from build123d import *

# Parameters (mm, degrees)
SKETCH1_W           = 76.72
SKETCH1_H           = 26.686
BOSS_EXTRUDE1_DEPTH = 15
SKETCH2_W           = 11
SKETCH2_H           = 5
CUT_EXTRUDE1_DEPTH  = 69.000448499
SKETCH3_R           = 1.5
CUT_EXTRUDE2_DEPTH  = 25
CUT_EXTRUDE3_DEPTH  = 3
CUT_EXTRUDE5_DEPTH  = 7
FILLET1_R           = 5


with BuildPart() as part:
    # Sketch1 → Boss-Extrude1 (new body)
    with BuildSketch(Plane.XY):
        with Locations((22.36, 8.343)):
            Rectangle(SKETCH1_W, SKETCH1_H)
        Polygon((0, 0), (0, 12), (3.02, 16.686), (5.22, 16.686), (8.24, 12), (8.24, 0), align=None, mode=Mode.SUBTRACT)
        Polygon((23.46, 16.686), (26.48, 12), (26.48, 0), (18.24, 0), (18.24, 12), (21.26, 16.686), align=None, mode=Mode.SUBTRACT)
        Polygon((41.7, 16.686), (44.72, 12), (44.72, 0), (36.48, 0), (36.48, 12), (39.5, 16.686), align=None, mode=Mode.SUBTRACT)
    extrude(amount=BOSS_EXTRUDE1_DEPTH)

    # Sketch2 → Cut-Extrude1 (cut, through all)
    with BuildSketch(Plane(origin=(0, -5, 0), x_dir=(-1, 0, 0), z_dir=(0, -1, 0))):
        with Locations((10.5, -12.5)):
            Rectangle(SKETCH2_W, SKETCH2_H)
        with Locations((-55.22, -12.5)):
            Rectangle(SKETCH2_W, SKETCH2_H)
    extrude(amount=-CUT_EXTRUDE1_DEPTH, mode=Mode.SUBTRACT)

    # Sketch3 → Cut-Extrude2 (cut)
    with BuildSketch(Plane.XY.offset(10)):
        with Locations((-10.5, 7.331502285)):
            Circle(SKETCH3_R)
        with Locations((55.22, 7.331502285)):
            Circle(SKETCH3_R)
    extrude(amount=-CUT_EXTRUDE2_DEPTH, mode=Mode.SUBTRACT)

    # Sketch4 → Cut-Extrude3 (cut)
    with BuildSketch(Plane.XY.offset(10)):
        Polygon((-10.5, 10.651266332), (-13.375, 8.991384309), (-13.375, 5.671620261), (-10.5, 4.011738237), (-7.625, 5.671620261), (-7.625, 8.991384309), align=None)
        Polygon((55.22, 10.651266332), (52.345, 8.991384309), (52.345, 5.671620261), (55.22, 4.011738237), (58.095, 5.671620261), (58.095, 8.991384309), align=None)
    extrude(amount=-CUT_EXTRUDE3_DEPTH, mode=Mode.SUBTRACT)

    # Sketch7 → Cut-Extrude5 (cut)
    with BuildSketch(Plane(origin=(0, 0, 0), x_dir=(-1, 0, 0), z_dir=(0, 0, -1))):
        Polygon((0, 0), (-12.36, 0), (-12.36, -5), (-32.36, -5), (-32.36, 0), (-44.72, 0), (-44.72, 16.686), (0, 16.686), align=None)
    extrude(amount=-CUT_EXTRUDE5_DEPTH, mode=Mode.SUBTRACT)

    # Fillet1
    # the kernel refuses this fillet: 5 mm, written as the material it adds along each edge
    with BuildSketch(Plane(origin=(49.72, -5, 10), x_dir=(0, 0, 1), z_dir=(0, 1, 0))) as fillet1_piece_1_section:
        with BuildLine():
            CenterArc((FILLET1_R, FILLET1_R), FILLET1_R, 180, 90)
            Line((0, FILLET1_R), (0, 0))
            Line((0, 0), (FILLET1_R, 0))
        make_face()
    fillet1_piece_1 = extrude(amount=26.686, mode=Mode.PRIVATE)
    fillet1_piece_1 = split(fillet1_piece_1, bisect_by=Plane(origin=(52.345, 0.855809372, 11.280904263), z_dir=(-1, 0, 0)), keep=Keep.TOP, mode=Mode.PRIVATE)
    fillet1_piece_1 = split(fillet1_piece_1, bisect_by=Plane(origin=(53.079309625, 5.247666401, 11.280904263), z_dir=(-0.5000000000000012, -0.866025403784438, 0)), keep=Keep.TOP, mode=Mode.PRIVATE)
    add(fillet1_piece_1)
    with BuildSketch(Plane(origin=(49.72, -5, 10), x_dir=(0, 0, 1), z_dir=(0, 1, 0))) as fillet1_piece_2_section:
        with BuildLine():
            CenterArc((FILLET1_R, FILLET1_R), FILLET1_R, 180, 90)
            Line((0, FILLET1_R), (0, 0))
            Line((0, 0), (FILLET1_R, 0))
        make_face()
    fillet1_piece_2 = extrude(amount=26.686, mode=Mode.PRIVATE)
    fillet1_piece_2 = split(fillet1_piece_2, bisect_by=Plane(origin=(52.345, 0.113882783, 10.103766802), z_dir=(1, 0, 0)), keep=Keep.TOP, mode=Mode.PRIVATE)
    fillet1_piece_2 = split(fillet1_piece_2, bisect_by=Plane(origin=(55.328155085, 3.94929487, 10.103766802), z_dir=(-0.5000000000000012, -0.866025403784438, 0)), keep=Keep.TOP, mode=Mode.PRIVATE)
    add(fillet1_piece_2)
    with BuildSketch(Plane(origin=(49.72, -5, 10), x_dir=(0, 0, 1), z_dir=(0, 1, 0))) as fillet1_piece_3_section:
        with BuildLine():
            CenterArc((FILLET1_R, FILLET1_R), FILLET1_R, 180, 90)
            Line((0, FILLET1_R), (0, 0))
            Line((0, 0), (FILLET1_R, 0))
        make_face()
    fillet1_piece_3 = extrude(amount=26.686, mode=Mode.PRIVATE)
    fillet1_piece_3 = split(fillet1_piece_3, bisect_by=Plane(origin=(50.660222367, 8.018677488, 10.86123456), z_dir=(0.5000000000000002, -0.8660254037844386, 0)), keep=Keep.TOP, mode=Mode.PRIVATE)
    fillet1_piece_3 = split(fillet1_piece_3, bisect_by=Plane(origin=(52.345, 7.331502285, 10.86123456), z_dir=(-1, 0, 0)), keep=Keep.TOP, mode=Mode.PRIVATE)
    fillet1_piece_3 = split(fillet1_piece_3, bisect_by=Plane(origin=(50.660222367, 6.644327081, 10.86123456), z_dir=(0.5000000000000012, 0.866025403784438, 0)), keep=Keep.TOP, mode=Mode.PRIVATE)
    add(fillet1_piece_3)
    with BuildSketch(Plane(origin=(49.72, -5, 10), x_dir=(0, 0, 1), z_dir=(0, 1, 0))) as fillet1_piece_4_section:
        with BuildLine():
            CenterArc((FILLET1_R, FILLET1_R), FILLET1_R, 180, 90)
            Line((0, FILLET1_R), (0, 0))
            Line((0, 0), (FILLET1_R, 0))
        make_face()
    fillet1_piece_4 = extrude(amount=26.686, mode=Mode.PRIVATE)
    fillet1_piece_4 = split(fillet1_piece_4, bisect_by=Plane(origin=(53.520712077, 9.670181993, 11.277716929), z_dir=(-0.5000000000000002, 0.8660254037844386, 0)), keep=Keep.TOP, mode=Mode.PRIVATE)
    fillet1_piece_4 = split(fillet1_piece_4, bisect_by=Plane(origin=(52.345, 14.819818281, 11.277716929), z_dir=(-1, 0, 0)), keep=Keep.TOP, mode=Mode.PRIVATE)
    add(fillet1_piece_4)
    with BuildSketch(Plane(origin=(49.72, -5, 10), x_dir=(0, 0, 1), z_dir=(0, 1, 0))) as fillet1_piece_5_section:
        with BuildLine():
            CenterArc((FILLET1_R, FILLET1_R), FILLET1_R, 180, 90)
            Line((0, FILLET1_R), (0, 0))
            Line((0, 0), (FILLET1_R, 0))
        make_face()
    fillet1_piece_5 = extrude(amount=26.686, mode=Mode.PRIVATE)
    fillet1_piece_5 = split(fillet1_piece_5, bisect_by=Plane(origin=(55.769242126, 10.968371422, 10.103260702), z_dir=(-0.5000000000000002, 0.8660254037844386, 0)), keep=Keep.TOP, mode=Mode.PRIVATE)
    fillet1_piece_5 = split(fillet1_piece_5, bisect_by=Plane(origin=(52.345, 15.561640812, 10.103260702), z_dir=(1, 0, 0)), keep=Keep.TOP, mode=Mode.PRIVATE)
    add(fillet1_piece_5)
    with BuildSketch(Plane(origin=(-5, -5, 10), x_dir=(-1, 0, 0), z_dir=(0, 1, 0))) as fillet1_piece_6_section:
        with BuildLine():
            CenterArc((FILLET1_R, FILLET1_R), FILLET1_R, 180, 90)
            Line((0, FILLET1_R), (0, 0))
            Line((0, 0), (FILLET1_R, 0))
        make_face()
    fillet1_piece_6 = extrude(amount=26.686, mode=Mode.PRIVATE)
    fillet1_piece_6 = split(fillet1_piece_6, bisect_by=Plane(origin=(-10.608155085, 3.94929487, 10.103766802), z_dir=(0.5000000000000003, -0.8660254037844387, 0)), keep=Keep.TOP, mode=Mode.PRIVATE)
    fillet1_piece_6 = split(fillet1_piece_6, bisect_by=Plane(origin=(-7.625, 0.113882783, 10.103766802), z_dir=(-1, 0, 0)), keep=Keep.TOP, mode=Mode.PRIVATE)
    add(fillet1_piece_6)
    with BuildSketch(Plane(origin=(-5, -5, 10), x_dir=(-1, 0, 0), z_dir=(0, 1, 0))) as fillet1_piece_7_section:
        with BuildLine():
            CenterArc((FILLET1_R, FILLET1_R), FILLET1_R, 180, 90)
            Line((0, FILLET1_R), (0, 0))
            Line((0, 0), (FILLET1_R, 0))
        make_face()
    fillet1_piece_7 = extrude(amount=26.686, mode=Mode.PRIVATE)
    fillet1_piece_7 = split(fillet1_piece_7, bisect_by=Plane(origin=(-8.359309625, 5.247666401, 11.280904263), z_dir=(0.5000000000000003, -0.8660254037844387, 0)), keep=Keep.TOP, mode=Mode.PRIVATE)
    fillet1_piece_7 = split(fillet1_piece_7, bisect_by=Plane(origin=(-7.625, 0.855809372, 11.280904263), z_dir=(1, 0, 0)), keep=Keep.TOP, mode=Mode.PRIVATE)
    add(fillet1_piece_7)
    with BuildSketch(Plane(origin=(-5, -5, 10), x_dir=(-1, 0, 0), z_dir=(0, 1, 0))) as fillet1_piece_8_section:
        with BuildLine():
            CenterArc((FILLET1_R, FILLET1_R), FILLET1_R, 180, 90)
            Line((0, FILLET1_R), (0, 0))
            Line((0, 0), (FILLET1_R, 0))
        make_face()
    fillet1_piece_8 = extrude(amount=26.686, mode=Mode.PRIVATE)
    fillet1_piece_8 = split(fillet1_piece_8, bisect_by=Plane(origin=(-5.940222366, 6.644327081, 10.861234561), z_dir=(-0.5000000000000003, 0.8660254037844387, 0)), keep=Keep.TOP, mode=Mode.PRIVATE)
    fillet1_piece_8 = split(fillet1_piece_8, bisect_by=Plane(origin=(-7.625, 7.331502285, 10.861234561), z_dir=(1, 0, 0)), keep=Keep.TOP, mode=Mode.PRIVATE)
    fillet1_piece_8 = split(fillet1_piece_8, bisect_by=Plane(origin=(-5.940222366, 8.018677488, 10.861234561), z_dir=(-0.49999999999999967, -0.8660254037844388, 0)), keep=Keep.TOP, mode=Mode.PRIVATE)
    add(fillet1_piece_8)
    with BuildSketch(Plane(origin=(-5, -5, 10), x_dir=(-1, 0, 0), z_dir=(0, 1, 0))) as fillet1_piece_9_section:
        with BuildLine():
            CenterArc((FILLET1_R, FILLET1_R), FILLET1_R, 180, 90)
            Line((0, FILLET1_R), (0, 0))
            Line((0, 0), (FILLET1_R, 0))
        make_face()
    fillet1_piece_9 = extrude(amount=26.686, mode=Mode.PRIVATE)
    fillet1_piece_9 = split(fillet1_piece_9, bisect_by=Plane(origin=(-7.625, 15.561640812, 10.103260702), z_dir=(-1, 0, 0)), keep=Keep.TOP, mode=Mode.PRIVATE)
    fillet1_piece_9 = split(fillet1_piece_9, bisect_by=Plane(origin=(-11.049242126, 10.968371422, 10.103260702), z_dir=(0.49999999999999967, 0.8660254037844388, 0)), keep=Keep.TOP, mode=Mode.PRIVATE)
    add(fillet1_piece_9)
    with BuildSketch(Plane(origin=(-5, -5, 10), x_dir=(-1, 0, 0), z_dir=(0, 1, 0))) as fillet1_piece_10_section:
        with BuildLine():
            CenterArc((FILLET1_R, FILLET1_R), FILLET1_R, 180, 90)
            Line((0, FILLET1_R), (0, 0))
            Line((0, 0), (FILLET1_R, 0))
        make_face()
    fillet1_piece_10 = extrude(amount=26.686, mode=Mode.PRIVATE)
    fillet1_piece_10 = split(fillet1_piece_10, bisect_by=Plane(origin=(-7.625, 14.819818281, 11.277716929), z_dir=(1, 0, 0)), keep=Keep.TOP, mode=Mode.PRIVATE)
    fillet1_piece_10 = split(fillet1_piece_10, bisect_by=Plane(origin=(-8.800712077, 9.670181993, 11.277716929), z_dir=(0.49999999999999967, 0.8660254037844388, 0)), keep=Keep.TOP, mode=Mode.PRIVATE)
    add(fillet1_piece_10)
    # the kernel refuses this fillet: 5 mm, written as the material it takes off along each edge
    with BuildSketch(Plane(origin=(60.72, -17.5, 10), x_dir=(0, 0, -1), z_dir=(0, 1, 0)), Plane(origin=(-16, -17.5, 10), x_dir=(1, 0, 0), z_dir=(0, 1, 0))) as fillet1_2_piece_1:
        with BuildLine():
            CenterArc((FILLET1_R, FILLET1_R), FILLET1_R, 180, 90)
            Line((0, FILLET1_R), (0, 0))
            Line((0, 0), (FILLET1_R, 0))
        make_face()
    extrude(amount=51.686, mode=Mode.SUBTRACT)
    with BuildSketch(Plane(origin=(73.22, 21.686, 10), x_dir=(0, 0, -1), z_dir=(-1, 0, 0)), Plane(origin=(-10, 21.686, 10), x_dir=(0, 0, -1), z_dir=(-1, 0, 0))) as fillet1_2_piece_2:
        with BuildLine():
            CenterArc((FILLET1_R, FILLET1_R), FILLET1_R, 180, 90)
            Line((0, FILLET1_R), (0, 0))
            Line((0, 0), (FILLET1_R, 0))
        make_face()
    extrude(amount=18.5, mode=Mode.SUBTRACT)
    with BuildSketch(Plane(origin=(73.22, -5, 10), x_dir=(0, 0, -1), z_dir=(-1, 0, 0)), Plane(origin=(-10, -5, 10), x_dir=(0, 0, -1), z_dir=(-1, 0, 0))) as fillet1_2_piece_3:
        with BuildLine():
            CenterArc((FILLET1_R, -FILLET1_R), FILLET1_R, 90, 90)
            Line((0, -FILLET1_R), (0, 0))
            Line((0, 0), (FILLET1_R, 0))
        make_face()
    extrude(amount=18.5, mode=Mode.SUBTRACT)
    with BuildSketch(Plane(origin=(-10, -5, 15), x_dir=(-0.8017442392976459, 0, 0.5976672776328307), z_dir=(-0.5976672776328307, 0, -0.8017442392976459))) as fillet1_2_piece_4:
        with BuildLine():
            CenterArc((5 + FILLET1_R, FILLET1_R), FILLET1_R, 180, 90)
            Line((5, FILLET1_R), (5, 0))
            Line((5, 0), (5 + FILLET1_R, 0))
        make_face()
    revolve(axis=Axis((-10, -5, 15), (0, 1, 0)), revolution_arc=233.296989237, mode=Mode.SUBTRACT)
    with BuildSketch(Plane(origin=(-10, 21.686, 15), x_dir=(0, 0, -1), z_dir=(-1, 0, 0))) as fillet1_2_piece_5:
        with BuildLine():
            CenterArc((5 + FILLET1_R, FILLET1_R), FILLET1_R, 180, 90)
            Line((5, FILLET1_R), (5, 0))
            Line((5, 0), (5 + FILLET1_R, 0))
        make_face()
    revolve(axis=Axis((-10, 21.686, 15), (0, -1, 0)), revolution_arc=233.296989237, mode=Mode.SUBTRACT)
    with BuildSketch(Plane(origin=(54.72, -5, 15), x_dir=(0, 0, -1), z_dir=(1, 0, 0))) as fillet1_2_piece_6:
        with BuildLine():
            CenterArc((5 + FILLET1_R, FILLET1_R), FILLET1_R, 180, 90)
            Line((5, FILLET1_R), (5, 0))
            Line((5, 0), (5 + FILLET1_R, 0))
        make_face()
    revolve(axis=Axis((54.72, -5, 15), (0, 1, 0)), revolution_arc=233.296989237, mode=Mode.SUBTRACT)
    with BuildSketch(Plane(origin=(54.72, 21.686, 15), x_dir=(0.8017442392976476, 0, 0.5976672776328285), z_dir=(0.5976672776328285, 0, -0.8017442392976476))) as fillet1_2_piece_7:
        with BuildLine():
            CenterArc((5 + FILLET1_R, FILLET1_R), FILLET1_R, 180, 90)
            Line((5, FILLET1_R), (5, 0))
            Line((5, 0), (5 + FILLET1_R, 0))
        make_face()
    revolve(axis=Axis((54.72, 21.686, 15), (0, -1, 0)), revolution_arc=233.296989237, mode=Mode.SUBTRACT)


solid = part.part
Read the model definition and answer for the solid it produces. Units are mm, in the model's axes. A direction names the side the tool comes from. Coordinates: 2 decimals unless noted, no trailing zeros. Loops run counter-clockwise (first coordinate to the right, second up) from the corner with the lowest first, then second, coordinate; pieces in that order, holes last. Notation, with made-up numbers: (-24.5, 11.5) -> (1.5, 11.5) arc R24 cw to (1.5, 31.5) -> close; hole circle Ø11 at (80, 22). An arc over 180 degrees is marked (long way). Write item = value, one per line. Start each with the question number.
1) Find the intervals of material crossed by L1, parallel to Y at x = -10.5, z = 4; L2, parallel to X at y = 8.5, z = 11.5; L3, parallel to Y at x = 23, z = 8.25, in increasing order. Write a range as from..to.
2) The part is cut by section A-A, the plane y = 12.75. Determine the outline of the cut face in (x, z), plus the area to 3 significant figures.
3) The mould has two halves that part along Y. Classify faces 1 (the face through (32.36, -3, 3)), 2 (the face through (52.345, 7, 9)), 3 (the face through (57, -4, 8)), 4 (the face through (37.97, 14.31, 10.94)): pulls with the +Y half, pulls with the -Y half, needs draft (parallel to the pull), parting line crosses it, or undercut.
4) For faces 5 (the face through (12.36, -2, 3)), 6 (the face through (44, 15, 7)), 7 (the face through (43.189, 14.376, 10.944)), 8 (the face through (-11.958, 4.853, 8.521)), 9 (the face through (16, 9, 15)), determine the directions among +Z, -Z, +X, -X, +Y, -Y from which every point of the face is accessible in a straight line to the end or side of a thin tool.
5) Given P1, Ø1.9, axis at y = 7.5, z = 7.5, coming from the +X side; P2, Ø11, axis at x = 28, y = 4, coming from the -Z side; P3, Ø6, axis at y = 13, z = 11, coming from the +X side; P4, Ø1.8, axis at x = 55.22, y = 7.33, coming from the +Z side, each flat-ended and moving along its own axis, determine where each tip first touches the part or whether it passes through.
6) The part is cut by section C-C, the plane z = 13.75. State how many separate pieces and enclosed holes the cut face has, plus the area to 3 significant figures.
7) The part is cut by section B-B, the plane z = 1.25. Determine the outline of the cut face in (x, y), plus the area to 3 significant figures.
Result:
q1.L1 = -5..5.83, 8.83..21.69
q1.L2 = -6.43..0, 8.24..18.24, 26.48..36.48, 44.72..51.15
q1.L3 = -5..0, 16.69..21.69
q2.outline = (-16, 0) -> (0, 0) -> (0, 7) -> (0.48, 7) -> (0.48, 15) -> (-5, 15) arc R5 cw to (-10, 10) -> (-11, 10) arc R5 ccw to (-16, 5) -> close; (7.76, 7) -> (18.72, 7) -> (18.72, 15) -> (7.76, 15) -> close; (26, 7) -> (36.96, 7) -> (36.96, 15) -> (26, 15) -> close; (44.24, 7) -> (44.72, 7) -> (44.72, 0) -> (60.72, 0) -> (60.72, 5) arc R5 ccw to (55.72, 10) -> (54.72, 10) arc R5 cw to (49.72, 15) -> (44.24, 15) -> close
q2.area = 553 mm²
q3.face_1 = needs draft
q3.face_2 = undercut
q3.face_3 = pulls with the -Y half
q3.face_4 = undercut
q4.face_5 = -Z, -Y
q4.face_6 = -Z
q4.face_7 = +Z, -Z
q4.face_8 = +Z
q4.face_9 = +Z, +X, -X, +Y, -Y
q5.P1 = 60.47
q5.P2 = 7
q5.P3 = 59.72
q5.P4 = through
q6.separate_pieces = 1
q6.enclosed_holes = 3
q6.area = 1,080 mm²
q7.outline = (-16, -5) -> (12.36, -5) -> (12.36, 0) -> (0, 0) -> (0, 16.69) -> (44.72, 16.69) -> (44.72, 0) -> (32.36, 0) -> (32.36, -5) -> (60.72, -5) -> (60.72, 21.69) -> (-16, 21.69) -> close; hole circle Ø3 at (-10.5, 7.33); hole circle Ø3 at (55.22, 7.33)
q7.area = 1,190 mm²
